Autodesk Inventor part; units mm, degrees
ref_plane "Work Plane1" through (0, 0, 0) normal (-0.7071068, 0, 0.7071068) x (0, -1, 0)
ref_plane "XZ Plane" through (0, 0, 0) normal (0, 1, 0) x (-1, 0, 0)
sketch "Sketch1" plane through (0, 0, 0) normal (1, 0, 0) x (0, 1, 0)
  line L0 (0, 0) -> (13.7625, 0)
  line L1 (13.7625, 0) -> (13.7625, 10.31875)
  line L2 (13.7625, 10.31875) -> (0, 10.31875)
  line L3 (0, 10.31875) -> (0, 0)
  line L4 (13.7625, 10.31875) -> (11.38125, 10.31875)
  line L5 (11.38125, 10.31875) -> (11.38125, 12.7)
  line L6 (11.38125, 12.7) -> (13.7625, 12.7)
  line L7 (13.7625, 12.7) -> (13.7625, 10.31875)
  line L8 (0, 10.31875) -> (2.38125, 10.31875)
  line L9 (2.38125, 10.31875) -> (2.38125, 12.7)
  line L10 (2.38125, 12.7) -> (0, 12.7)
  line L11 (0, 12.7) -> (0, 10.31875)
  line L12 (13.7625, 4.2) -> (0, 4.2)
  line L13 (0, 4.2) -> (0, 0)
  line L14 (0, 0) -> (13.7625, 0)
  line L15 (13.7625, 0) -> (13.7625, 4.2)
  point P0 (0, 4.2)
  dimension "d1" = 10.31875
  dimension "d2" = 2.38125
  dimension "d3" = 2.38125
  dimension "d4" = 12.7
  dimension "d5" = 4.2
  dimension "d29" = 9
revolve "Revolution1" add sketch "Sketch1" angle 360 about axis through (0, 0, 0) along (0, 1, 0) contours L3 L2 L1 L12 | L11 L10 L9 L2 | L2 L5 L6 L7
sketch "Sketch2" plane through (0, 2.38125, 0) normal (0, 1, 0) x (1, 0, 0)
  circle A0 centre (0, 0) radius 4.2
  circle A1 centre (0, 0) radius 6.2
  line L0 (4.2, 0) -> (6.2, 0)
  line L1 (0, 4.2) -> (0, 6.2)
  circle A2 centre (0, 0) radius 10.31875
  line L2 (0, 6.2) -> (-9.425317, 6.2)
  line L3 (-9.425317, 6.2) -> (-9.425317, 4.2)
  line L4 (-9.425317, 4.2) -> (0, 4.2)
  line L5 (0, 4.2) -> (0, 6.2)
  line L6 (10.31875, 0) -> (8.81875, 0)
  arc A3 (8.81875, 0) -> (-10.31875, 0) centre (-0.75, 0) ccw
  dimension "d7" = 2
  dimension "d30" = 1.5
sketch "Sketch2 outline for Extrusion1" plane through (0, 2.38125, 0) normal (0, 1, 0) x (1, 0, 0)
  arc A0 (-10.31875, 0) -> (8.81875, 0) centre (-0.75, 0) cw
  arc A1 (10.31875, 0) -> (-10.31875, 0) centre (0, 0) ccw
  line L0 (8.81875, 0) -> (10.31875, 0)
extrude "Extrusion1" cut sketch "Sketch2 outline for Extrusion1" along normal up to surface (9 mm away)
ref_plane "Work Plane1" through (0, 0, 0) normal (-0.7071068, 0, 0.7071068) x (0, -1, 0)
sketch "Sketch3" plane through (0, 0, 0) normal (-0.7071068, 0, 0.7071068) x (0, -1, 0)
  line L0 (0, 0) -> (-13.7625, 0) construction
  line L1 (-13.7625, 4.2) -> (-13.7625, -4.2)
  circle A0 centre (-6.88125, 0) radius 1.651
  dimension "d12" = 3.302
extrude "Extrusion2" cut sketch "Sketch3" against normal through all
chamfer "Chamfer1" distance 0.5 angle 45 2 edges at (0, 0, -4.2) (0, 13.7625, -4.2)
chamfer "Chamfer2" distance 0.5 angle 45 1 edges at (6.7558, 8.4269, -5.935)
chamfer "Chamfer3" distance 0.5 angle 45 2 edges at (0, 13.7625, -12.7) (0, 0, -12.7)
fillet "Fillet3" radius 1 1 edges at (10.3188, 6.8812, 0)
equation "\"d3\" = d2"
properties part number "Spring Spool" material "Nylon 6/6"
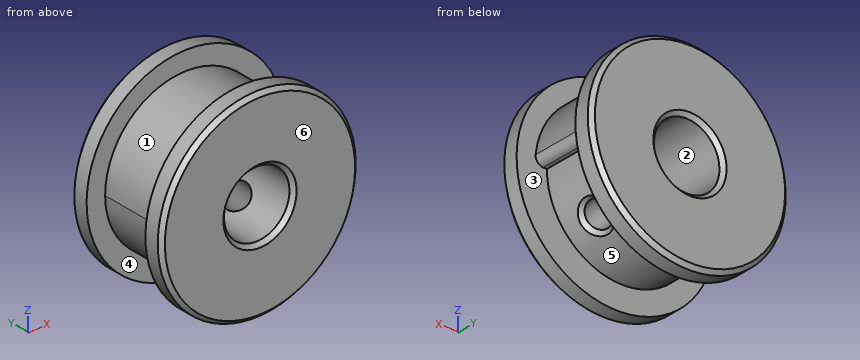
Source: CAD feature listing. Evaluate the final solid. Frame: model axes, mm. Face numbers are marked on the shaded views. A direction names the side the tool comes from. Give positions to 0.01 mm unless a question says otherwise; leave off trailing zeros. Write each loop counter-clockwise with the first axis right and the second up, starting at its lowest first coordinate (ties: lowest second). Pieces come first, ordered by that corner, then holes. Notation, with made-up numbers: (-5, -17) -> (48, -17) arc R28 ccw to (48, 13) -> close; hole circle Ø11 at (12.25, 56.25). An arc over 180 degrees is marked (long way). Return JSON: item names as keys, results as strings. Group by question number.
1. Section B-B, the plane x = 0. Output: boundary loops of the cut face in (y, z).
2. Section A-A, the plane y = 12.75. Output: boundary loops of the cut face in (x, z).
3. Mould query, pull axis Z, two halves, no side actions, for the marked faces 1, 2 and 3. Classes: +Z half, -Z half, draft (parallel to the pull), parting line (faces both ways), or undercut.
4. Pin query (flat end, axial travel): pin 1 Ø4 at (x, z) = (0, -1) entering from -Y; pin 2 Ø1.5 at (x, y) = (0.5, 8) entering from +Z; pin 3 Ø8 at (x, y) = (4.5, 4) entering from +Z; pin 4 Ø8 at (y, z) = (3.5, -6) entering from +X. Return the tip coordinate at first contact, or that it passes through.
5. Access query for the marked faces 4, 5 and 6. Directions: +Z, -Z, +X, -X, +Y, -Y. A direction counts if a zero-diameter tool reaches every point of the face in a straight line with its end or side. Return the directions, or none.
6. Material intervals for line 1 (Y direction, x = -10.5, z = 1.25); line 2 (Z direction, x = -1, y = 5.5); line 3 (X direction, y = 1.75, z = -3.25), sorted ascending. Write a range as from..to.
Determined:
{
 "1": {"outline": "(0, -12.2) -> (0.5, -12.7) -> (2.38, -12.7) -> (2.38, -9.54) -> (11.38, -9.54) -> (11.38, -12.7) -> (13.26, -12.7) -> (13.76, -12.2) -> (13.76, -4.7) -> (13.26, -4.2) -> (0.5, -4.2) -> (0, -4.7) -> close; (0, 4.7) -> (0.5, 4.2) -> (13.26, 4.2) -> (13.76, 4.7) -> (13.76, 12.2) -> (13.26, 12.7) -> (11.38, 12.7) -> (11.38, 10.32) -> (2.38, 10.32) -> (2.38, 12.7) -> (0.5, 12.7) -> (0, 12.2) -> close"},
 "2": {"outline": "circle Ø25.4 at (0, 0); hole circle Ø8.4 at (0, 0)"},
 "3": {"face 1": "+Z half", "face 2": "undercut", "face 3": "draft"},
 "4": {"pin 1": "passes through", "pin 2": "stops at z = 10.32", "pin 3": "stops at z = 12.67", "pin 4": "stops at x = 12.52"},
 "5": {"face 4": "none", "face 5": "-Z", "face 6": "+Z, -Z, +X, -X, -Y"},
 "6": {"line 1": "y = 0..2.38, 11.38..13.76", "line 2": "z = -9.57..-4.08, 4.08..10.27", "line 3": "x = -12.28..-2.66, 2.66..12.28"}
}
